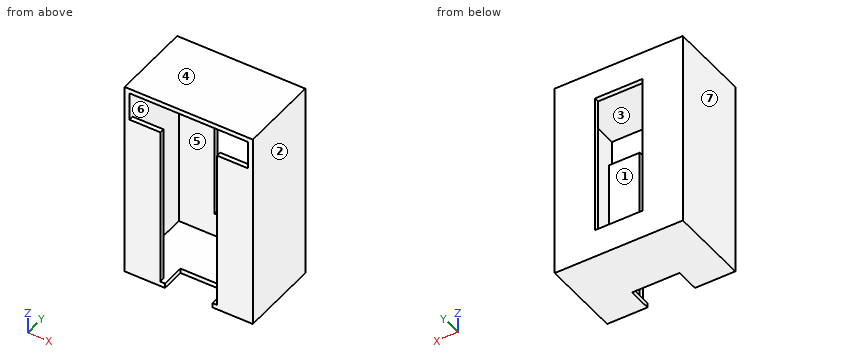
from build123d import *

# Parameters (mm, degrees)
F0_W      = 54
F0_H      = 84
F1_DEPTH  = 34
F2_T      = -2
F3_W      = 20
F3_H      = 60
F4_DEPTH  = 25
F5_W      = 15
F5_H      = 70
F6_DEPTH  = 2
F7_W      = 15
F7_H      = 70
F8_DEPTH  = 2
F9_W      = 10
F9_H      = 2
F10_DEPTH = 10


with BuildPart() as f1:
    # F0 (on Front) → F1 (new body)
    with BuildSketch(Plane.XZ):
        Rectangle(F0_W, F0_H)
    extrude(amount=F1_DEPTH)

    # F2
    f2_openings = [f1.faces().sort_by_distance(p)[0] for p in [
        (0, -34, 0),
    ]]
    offset(amount=F2_T, openings=f2_openings)

    # F3 (on face) → F4 (cut)
    with BuildSketch(Plane.XZ.offset(2)):
        Rectangle(F3_W, F3_H)
    extrude(amount=-F4_DEPTH, mode=Mode.SUBTRACT)

    # F5 (on face) → F6 (join)
    with BuildSketch(Plane.XZ.offset(34)):
        with Locations((-19.5, -7)):
            Rectangle(F5_W, F5_H)
    extrude(amount=-F6_DEPTH)

    # F7 (on face) → F8 (join)
    with BuildSketch(Plane.XZ.offset(34)):
        with Locations((19.5, -7)):
            Rectangle(F7_W, F7_H)
    extrude(amount=-F8_DEPTH)

    # F9 (on face) → F10 (cut)
    with BuildSketch(Plane.XZ.offset(34)):
        with Locations((-5, -41)):
            Rectangle(F9_W, F9_H)
        with Locations((5, -41)):
            Rectangle(F9_W, F9_H)
    extrude(amount=-F10_DEPTH, mode=Mode.SUBTRACT)


solid = f1.part
CAD build for the part. Positions are in the model's coordinates, mm. Face numbers are marked on the shaded views. A direction names the side the tool comes from. Round coordinates to 2 decimals unless told otherwise and drop trailing zeros. Loops run counter-clockwise (first coordinate to the right, second up) from the corner with the lowest first, then second, coordinate; pieces in that order, holes last. Notation, with made-up numbers: M 62.25,28 L 121.25,28 A30 cw 121.25,58 Z; hole C 28,78 d8. An arc over 180 degrees is marked long. One line per question, with ' | ' between items. Start each with the question number.
Item 1: Cut at C-C, the plane y = -4.5. Write the cut outline in (x, z), plus the area to 3 significant figures.
Item 2: Which spindle directions (+Z, -Z, +X, -X, +Y, -Y) get a long thin tool onto all of the face, cutting with end or side? Do the marked faces 1, 2 and 3. Say none if no direction does.
Item 3: Cut at B-B, the plane z = -12. Write the cut outline in (x, y), plus the area to 3 significant figures.
Item 4: Cut at A-A, the plane x = 3. Write the cut outline in (y, z).
Item 5: Wall check: line 1 (Y direction, x = 14, z = 0); line 2 (Z direction, x = 1, y = -8.5); line 3 (X direction, y = -27, z = 6). Give the ranges that are in metal, low to high.
Item 6: Cut at D-D, the plane y = -30.5. Write the cut outline in (x, z).
Item 7: Pin check, flat tip, straight feed: pin 1 Ø2 at (x, z) = (0.5, -41) entering from -Y. Stop position of the tip, or through.
Item 8: Two-plate mould, pull along Z, no slides. Class the marked faces 4, 5, 6 and 7: pulls with the +Z half, pulls with the -Z half, needs draft (parallel to the pull), parting line crosses it, or undercut.
Responses:
1) outline: M -27,-42 L 27,-42 L 27,42 L -27,42 Z; hole M -25,-40 L 25,-40 L 25,40 L -25,40 Z | area: 536 mm²
2) face 1: none | face 2: +Z, -Z, +X, +Y, -Y | face 3: -Y
3) outline: M -27,-34 L -12,-34 L -12,-32 L -25,-32 L -25,-2 L -10,-2 L -10,0 L -27,0 Z; M 10,-2 L 25,-2 L 25,-32 L 12,-32 L 12,-34 L 27,-34 L 27,0 L 10,0 Z | area: 248 mm²
4) outline: M -34,40 L -2,40 L -2,30 L 0,30 L 0,42 L -34,42 Z; M -24,-42 L 0,-42 L 0,-30 L -2,-30 L -2,-40 L -24,-40 Z
5) line 1: y = -34 to -32, -2 to 0 | line 2: z = -42 to -40, 40 to 42 | line 3: x = -27 to -25, 25 to 27
6) outline: M -27,-42 L -10,-42 L -10,-40 L -25,-40 L -25,40 L 25,40 L 25,-40 L 10,-40 L 10,-42 L 27,-42 L 27,42 L -27,42 Z
7) pin 1: stops at y = -24
8) face 4: pulls with the +Z half | face 5: undercut | face 6: undercut | face 7: needs draft
